Can you work these out from the drawing? Everything is in mm from the part's minimum corner. Give positions to 0.01 mm unless a question says otherwise; leave off trailing zeros. Write each loop counter-clockwise with the first axis right and the second up, starting at its lowest first coordinate (ties: lowest second). Pieces come first, ordered by that corner, then holes. Notation, with made-up numbers: (27.25, 53.25) -> (59.25, 53.25) arc R19 ccw to (59.25, 58.25) -> close; hole circle Ø8 at (20.5, 73). An arc over 180 degrees is marked (long way). Use one line per item in the form item = value.
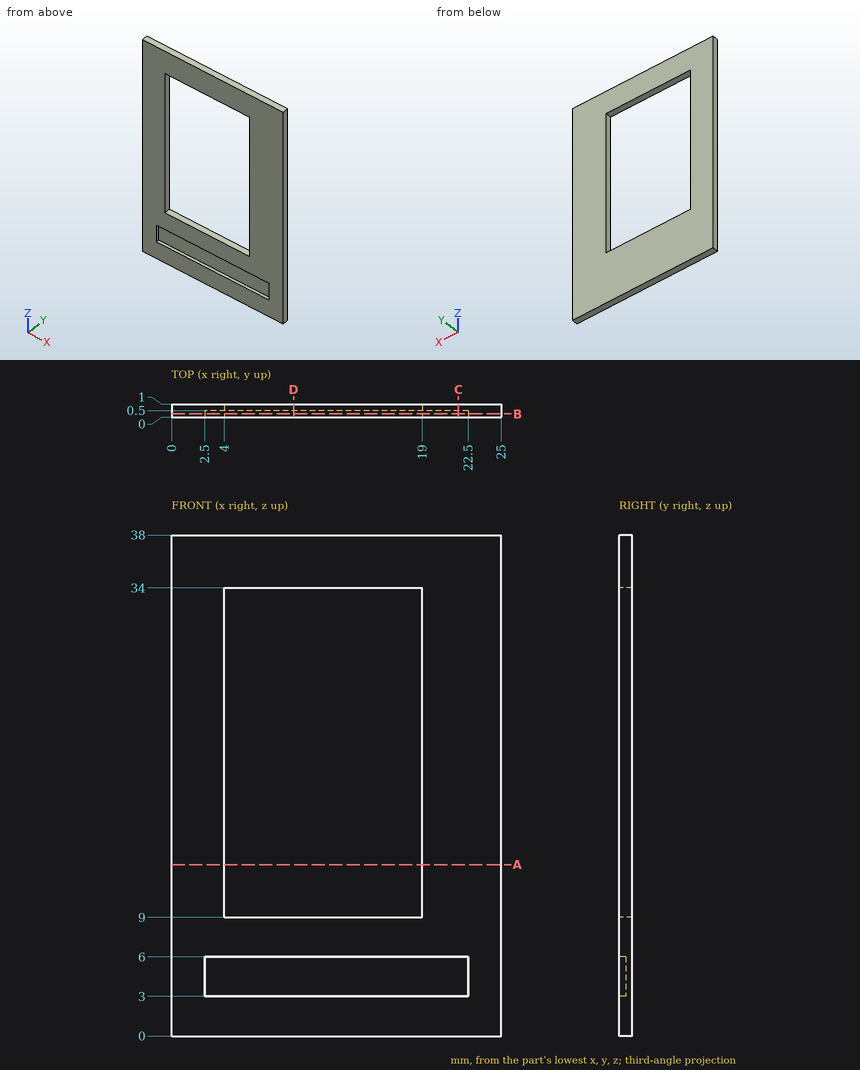
Q1. I want a section at A-A, the plane z = 13. Write out the boundary of the cut face in (x, y), and give its area (3 significant figures).
Result set:
outline = (0, 0) -> (4, 0) -> (4, 1) -> (0, 1) -> close; (19, 0) -> (25, 0) -> (25, 1) -> (19, 1) -> close
area = 10.0 mm2
Q2. I want a section at B-B, the plane y = 0.25. Write out the boundary of the cut face in (x, z), and give its area (3 significant figures).
Result set:
outline = (0, 0) -> (25, 0) -> (25, 38) -> (0, 38) -> close; hole (2.5, 3) -> (22.5, 3) -> (22.5, 6) -> (2.5, 6) -> close; hole (4, 9) -> (19, 9) -> (19, 34) -> (4, 34) -> close
area = 515 mm2
Q3. Will this pin go through, and if not, where does the flat tip stop? pin 1 Ø1.5 at (x, z) = (14, 4.5) entering from -Y.
Result set:
pin_1 = 0.5
Q4. If I drill on line 1 along Z through (x, y) = (12.5, 0.15); line 2 along Z through (x, y) = (7.75, 0.7); line 3 along X through (y, z) = (0.7, 31), over which ranges is the centre line in solid material (lowest first)? Write a range as from..to.
Result set:
line_1 = 0..3, 6..9, 34..38
line_2 = 0..9, 34..38
line_3 = 0..4, 19..25
Q5. I want a section at C-C, the plane x = 21.75. Write out the boundary of the cut face in (y, z).
Result set:
outline = (0, 0) -> (1, 0) -> (1, 38) -> (0, 38) -> (0, 6) -> (0.5, 6) -> (0.5, 3) -> (0, 3) -> close
Q6. I want a section at D-D, the plane x = 9.25. Write out the boundary of the cut face in (y, z).
Result set:
outline = (0, 0) -> (1, 0) -> (1, 9) -> (0, 9) -> (0, 6) -> (0.5, 6) -> (0.5, 3) -> (0, 3) -> close; (0, 34) -> (1, 34) -> (1, 38) -> (0, 38) -> close
